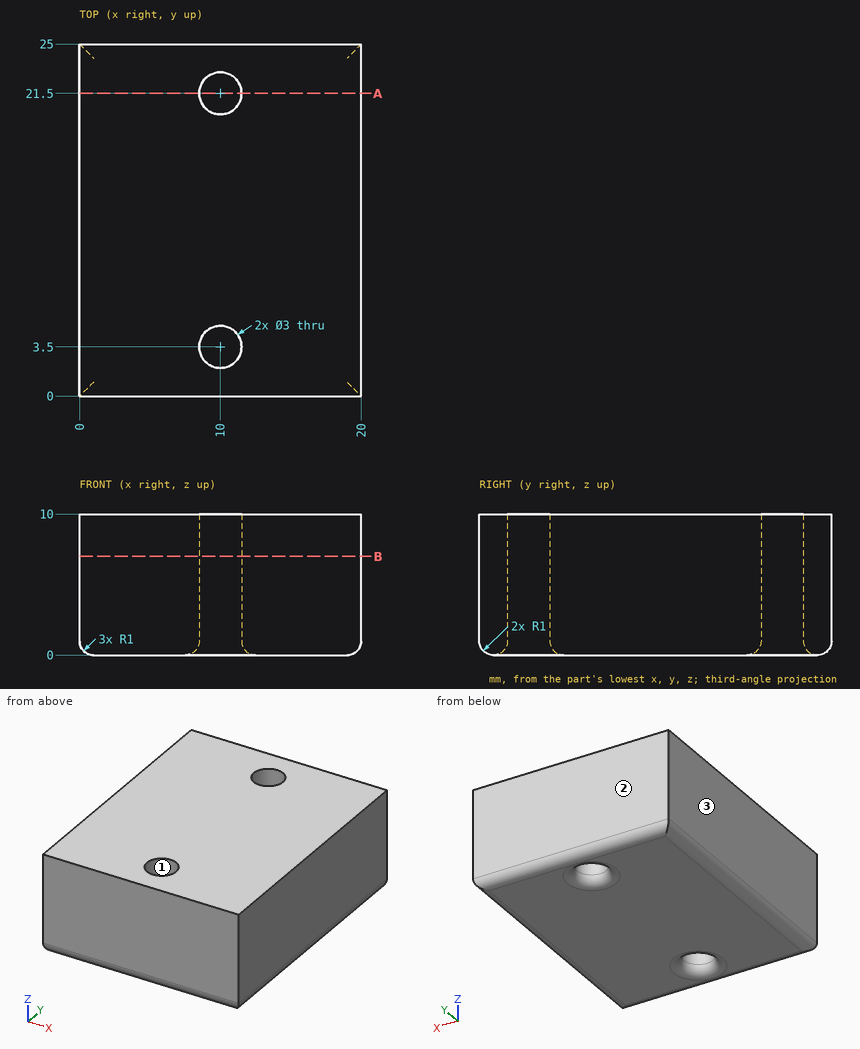
Here's the drawing with two shaded views (mm, measured from the low corner). I have some questions. Round coordinates to 2 decimals unless told otherwise and drop trailing zeros. Loops run counter-clockwise (first coordinate to the right, second up) from the corner with the lowest first, then second, coordinate; pieces in that order, holes last. Notation, with made-up numbers: M -29,-29.5 L 0,-29.5 A18 cw 0,-2.5 Z; hole C 45,69.25 d2. An arc over 180 degrees is marked long. Put each result on its own line as item: value.
Q1. I need wall thicknesses on probe 1 along Y at (x, z) = (10, 3.5); probe 2 along X at (y, z) = (21.5, 6.5); probe 3 along Y at (x, z) = (8.75, 5.5). Which ranges of each line are inside material? Lowest first, please.
Check result:
probe 1: 0 to 2, 5 to 20, 23 to 25
probe 2: 0 to 8.5, 11.5 to 20
probe 3: 0 to 2.67, 4.33 to 20.67, 22.33 to 25
Q2. Imagine slicing it at A-A (y = 21.5). Write out the boundary of the cut face in (x, z), then the cut area to 3 significant figures.
Check result:
outline: M 0,1 A1 ccw 1,0 L 7.5,0 A1 ccw 8.5,1 L 8.5,10 L 0,10 Z; M 11.5,1 A1 ccw 12.5,0 L 19,0 A1 ccw 20,1 L 20,10 L 11.5,10 Z
area: 169 mm2
Q3. For pin 1 (3 mm diameter, centred on y = 16, z = 7.5, fed in from -X), with a flat end and sliding along its axis, tell me the tip position at first contact or that it passes through.
Check result:
pin 1: x = 0
Q4. Imagine slicing it at B-B (z = 7). Write out the boundary of the cut face in (x, y).
Check result:
outline: M 0,0 L 20,0 L 20,25 L 0,25 Z; hole C 10,3.5 d3; hole C 10,21.5 d3
Q5. Thinking about a two-plate mould opening in Y: for the marked faces 1, 2 and 3, which applies, released by +Y, released by -Y, zero draft, split by the parting line, or undercut?
Check result:
face 1: undercut
face 2: released by +Y
face 3: zero draft
